Here's how the part is built. I have some questions about the finished solid (model axes, mm). A direction names the side the tool comes from. Round coordinates to 2 decimals unless told otherwise and drop trailing zeros. Loops run counter-clockwise (first coordinate to the right, second up) from the corner with the lowest first, then second, coordinate; pieces in that order, holes last. Notation, with made-up numbers: M 72,60.5 L 88,60.5 A37 ccw 88,97.5 Z; hole C 66.5,76.25 d6. An arc over 180 degrees is marked long. Answer as a JSON object with one key per item and string values.
Autodesk Inventor part; units mm, degrees
ref_plane "YZ Plane" through (0, 0, 0) normal (1, 0, 0) x (0, 1, 0)
ref_plane "XZ Plane" through (0, 0, 0) normal (0, 1, 0) x (-1, 0, 0)
ref_plane "XY Plane" through (0, 0, 0) normal (0, 0, 1) x (1, 0, 0)
sketch "スケッチ1" plane through (0, 0, 0) normal (1, 0, 0) x (0, 1, 0)
  line L0 (0, 0) -> (1.25, 0) construction
  line L1 (2.25, 0) -> (2.25, 2.2)
  line L2 (1.95, 2.5) -> (1.1547, 2.5)
  line L3 (0, 2.5) -> (0, 1.8333) construction
  line L4 (1.25, 0) -> (1.25, -8)
  line L5 (1.25, -8) -> (0, -8)
  line L6 (0, -8) -> (0, 0)
  line L7 (1.25, 0) -> (2.25, 0)
  line L8 (1.1547, 2.5) -> (0.5774, 1.5) construction
  line L9 (0.5774, 1.5) -> (-0.5774, 1.5) construction
  line L10 (-0.5774, 1.5) -> (-1.1547, 2.5) construction
  line L11 (-1.1547, 2.5) -> (-0.5774, 3.5) construction
  line L12 (-0.5774, 3.5) -> (0.5774, 3.5) construction
  line L13 (0.5774, 3.5) -> (1.1547, 2.5) construction
  line L14 (1.1547, 2.5) -> (0, 1.8333)
  line L15 (1.1547, 2.5) -> (0, 2.5) construction
  line L16 (0, 1.8333) -> (0, 0)
  arc A0 (2.25, 2.2) -> (1.95, 2.5) centre (1.95, 2.2) ccw
  dimension "d0" = 2
  dimension "d1" = 4.5
  dimension "d2" = 2.5
  dimension "d3" = 8
  dimension "d4" = 2.5
  dimension "d6" = 0.3
  dimension "d11" = 30
revolve "回転1" add sketch "スケッチ1" angle 360 about axis through (0, 0, 1.8333) along (0, 0, -1)
sketch "スケッチ2" plane through (0, 0, 2.5) normal (0, 0, 1) x (1, 0, 0)
  line L0 (1.1547, 0) -> (0.5774, -1)
  line L1 (0.5774, -1) -> (-0.5774, -1)
  line L2 (-0.5774, -1) -> (-1.1547, 0)
  line L3 (-1.1547, 0) -> (-0.5774, 1)
  line L4 (-0.5774, 1) -> (0.5774, 1)
  line L5 (0.5774, 1) -> (1.1547, 0)
  point P0 (0, 0)
  point P1 (0, 0)
  dimension "d8" = 2
extrude "押し出し1" cut sketch "スケッチ2" against normal blind 1
chamfer "面取り1" distance 0.25 angle 45 1 edges at (0, -1.25, -8)
properties part number "10_054_CAP_BOLT_M2_5X8_R1" material "鋼、炭素鋼"
Item 1: I want a section at A-A on x = 0. List the corners of the cut face in (y, z) for me.
Solution:
{"outline": "M -2.25,0 L -1.25,0 L -1.25,-7.75 L -1,-8 L 1,-8 L 1.25,-7.75 L 1.25,0 L 2.25,0 L 2.25,2.2 A0.3 ccw 1.95,2.5 L 1.15,2.5 L 1,2.41 L 1,1.5 L -1,1.5 L -1,2.41 L -1.15,2.5 L -1.95,2.5 A0.3 ccw -2.25,2.2 Z"}
Item 2: For faces 1 (the face through (-2.23, -0.29, 1.12)), 2 (the face through (0.87, -0.49, 2.01)), 3 (the face through (-1, 1, 0)), which set-ups out of +Z, -Z, +X, -X, +Y, -Y let a thin tool reach every point of the face, with its end or its side?
Solution:
{"face 1": "+Z, -Z", "face 2": "+Z", "face 3": "-Z"}
Item 3: We'd pull the mould along Y, two halves only. Please class faces 4 (the face through (-1, 1, 2.5)), 5 (the face through (0, -1, 2)), 6 (the face through (-1.22, -0.27, -3.93)): +Y half, -Y half, draft (parallel to the pull), parting line (faces both ways), or undercut.
Solution:
{"face 4": "draft", "face 5": "undercut", "face 6": "parting line"}
Item 4: I want a section at B-B on z = -4. List the corners of the cut face in (x, y) for me.
Solution:
{"outline": "C 0,0 d2.5"}
Item 5: If I drill on L1, parallel to Z at x = 0, y = 1.8; L2, parallel to Z at x = 0.25, y = 0.85; L3, parallel to X at y = 0.7, z = 0.75, over which ranges is the centre line in solid material (lowest first)? Write a range as from..to.
Solution:
{"L1": "z = 0..2.5", "L2": "z = -8..1.5", "L3": "x = -2.14..2.14"}
Item 6: For P1, Ø0.8, axis at x = 0.5, z = 2, coming from the +Y side; P2, Ø0.6, axis at x = -0.5, y = 0, coming from the +Z side; P3, Ø1.5, axis at x = 0, z = -1, coming from the +Y side, each with a flat end and sliding along its axis, tell me the tip position at first contact or that it passes through.
Solution:
{"P1": "stops at y = 2.25", "P2": "stops at z = 1.5", "P3": "stops at y = 1.25"}
